Check sheet for the modelled part. Datum: model origin and axes. Units: mm. A direction names the side the tool comes from. Round coordinates to 2 decimals unless told otherwise and drop trailing zeros. Write each loop counter-clockwise with the first axis right and the second up, starting at its lowest first coordinate (ties: lowest second). Pieces come first, ordered by that corner, then holes.
Item 1: Go/stop test with flat-tipped pins: pin 1 Ø1.8 at (x, z) = (0, -8) entering from +Y; pin 2 Ø2.5 at (x, z) = (9.5, 0) entering from -Y; pin 3 Ø4 at (x, y) = (-10, 8) entering from -Z. Record where each tip stops, or that it passes through.
Item 2: Material ranges on line 1 (Z direction, x = 0, y = 2.85); line 2 (Y direction, x = -10, z = -2.25); line 3 (X direction, y = 1.6, z = -8), recorded low to high.
Item 3: Cross-section at B-B on y = 19.5. Enter the section's corners in (x, z), plus the area to 3 significant figures.
Item 4: Cross-section at C-C on y = 10. Enter the section's corners in (x, z).
Item 5: Release check for a two-part mould opening along Z. For faces 3 (the flat face through (5, 0, 2)), 4 (the cylindrical face through (-0.54, 23.66, 2.44)), 5 (the conical face through (-0.12, 5.745, 8.231)), 6 (the cylindrical face through (-11, 3, 0)) record: +Z half, -Z half, draft (parallel to the pull), parting line (faces both ways), or undercut.
Item 6: Cross-section at A-A on y = 2.5. Enter the section's corners in (x, z), plus the area to 3 significant figures.
Item 7: Tool access check on faces 1 (the flat face through (0, -2, 0)), 2 (the cylindrical face through (-0.325, 2.535, 9.464)). Record the directions out of +Z, -Z, +X, -X, +Y, -Y that give a thin tool (end or side, any length) a straight path to the whole face; none if there is none.
from build123d import *

# Parameters (mm, degrees)
SKETCH1_R                    = 14.2
BOSS_EXTRUDE1_DEPTH          = 17
SKETCH2_R                    = 2.5
BOSS_EXTRUDE2_DEPTH          = 13.5
CHAMFER1_SIZE                = 2
CHAMFER1_SIZE2               = 1.154700538
F_3_0_3_DIAMETER_HOLE1_D     = 3
F_3_0_3_DIAMETER_HOLE1_DEPTH = 5
F_3_0_3_DIAMETER_HOLE1_TIP   = 0.901290929
CHAMFER3_SIZE                = 3
CHAMFER3_SIZE2               = 1.732050808
SKETCH6_R                    = 5
BOSS_EXTRUDE3_DEPTH          = 2


with BuildPart() as part:
    # Sketch1 → Boss-Extrude1 (new body)
    with BuildSketch(Plane(origin=(0, 0, 0), x_dir=(1, 0, 0), z_dir=(0, 1, 0))):
        Circle(SKETCH1_R)
    extrude(amount=BOSS_EXTRUDE1_DEPTH)

    # Sketch2 → Boss-Extrude2 (add)
    with BuildSketch(Plane(origin=(0, 17, 0), x_dir=(1, 0, 0), z_dir=(0, 1, 0))):
        Circle(SKETCH2_R)
    extrude(amount=BOSS_EXTRUDE2_DEPTH)

    # Chamfer1
    chamfer1_edges = [part.edges().sort_by_distance(p)[0] for p in [
        (-14.2, 17, 0),
    ]]
    chamfer1_side = [part.faces().sort_by_distance(p)[0] for p in [
        (-14.2, 8.5, 0),
    ]]
    chamfer(chamfer1_edges, length=CHAMFER1_SIZE, length2=CHAMFER1_SIZE2, reference=chamfer1_side[0])

    # Ø3.0 (3) Diameter Hole1
    with Locations(Plane(origin=(0, 0, 0), x_dir=(-1, 0, 0), z_dir=(0, -1, 0))):
        with Locations((0, -8), (-9.5, 0), (0, 8), (9.5, 0)):
            Hole(F_3_0_3_DIAMETER_HOLE1_D / 2, depth=F_3_0_3_DIAMETER_HOLE1_DEPTH)
            with Locations((0, 0, -(F_3_0_3_DIAMETER_HOLE1_DEPTH + F_3_0_3_DIAMETER_HOLE1_TIP / 2))):  # 118° drill point
                Cone(0, F_3_0_3_DIAMETER_HOLE1_D / 2, F_3_0_3_DIAMETER_HOLE1_TIP, mode=Mode.SUBTRACT)

    # Chamfer3
    chamfer3_edges = [part.edges().sort_by_distance(p)[0] for p in [
        (-14.2, 0, 0),
    ]]
    chamfer3_side = [part.faces().sort_by_distance(p)[0] for p in [
        (0, 0, 0),
    ]]
    chamfer(chamfer3_edges, length=CHAMFER3_SIZE, length2=CHAMFER3_SIZE2, reference=chamfer3_side[0])

    # Sketch6 → Boss-Extrude3 (add)
    with BuildSketch(Plane.XZ):
        Circle(SKETCH6_R)
    extrude(amount=BOSS_EXTRUDE3_DEPTH)


solid = part.part
Response values:
1. pin 1: stops at y = 17
1. pin 2: stops at y = 5.15
1. pin 3: stops at z = -11.73
2. line 1: z = -14.2 to -9.5, -6.5 to 6.5, 9.5 to 14.2
2. line 2: y = 0 to 17
2. line 3: x = -11.45 to -1.5, 1.5 to 11.45
3. outline: circle Ø5 at (0, 0)
3. area: 19.6 mm2
4. outline: circle Ø28.4 at (0, 0)
5. face 3: draft
5. face 4: parting line
5. face 5: undercut
5. face 6: undercut
6. outline: circle Ø28.4 at (0, 0); hole circle Ø3 at (-9.5, 0); hole circle Ø3 at (0, -8); hole circle Ø3 at (0, 8); hole circle Ø3 at (9.5, 0)
6. area: 605 mm2
7. face 1: +Z, -Z, +X, -X, -Y
7. face 2: -Y
